```python
from build123d import *

# Parameters (mm, degrees)
SKETCH2_W           = 45
SKETCH2_H           = 10
BOSS_EXTRUDE1_DEPTH = 40
SKETCH4_W           = 45
SKETCH4_H           = 10
BOSS_EXTRUDE2_DEPTH = 10
SKETCH8_W           = 45
SKETCH8_H           = 10
BOSS_EXTRUDE3_DEPTH = 20
SKETCH9_R           = 1.45
CUT_EXTRUDE2_DEPTH  = 20
SKETCH10_W          = 45
SKETCH10_H          = 0.626165357
CUT_EXTRUDE3_DEPTH  = 2
SKETCH11_W          = 19
SKETCH11_H          = 42.671327575
BOSS_EXTRUDE4_DEPTH = 1.5
SKETCH12_W          = 3
SKETCH12_H          = 27.286335608
CUT_EXTRUDE6_DEPTH  = 10
SKETCH13_W          = 13
SKETCH13_H          = 22
BOSS_EXTRUDE5_DEPTH = 1


with BuildPart() as part:
    # Sketch2 → Boss-Extrude1 (new body)
    with BuildSketch(Plane(origin=(0, 0, 0), x_dir=(1, 0, 0), z_dir=(0, 1, 0))):
        Rectangle(SKETCH2_W, SKETCH2_H)
    extrude(amount=BOSS_EXTRUDE1_DEPTH)

    # Sketch4 → Boss-Extrude2 (add)
    with BuildSketch(Plane(origin=(0, 40, 0), x_dir=(1, 0, 0), z_dir=(0, 1, 0))):
        Rectangle(SKETCH4_W, SKETCH4_H)
    extrude(amount=BOSS_EXTRUDE2_DEPTH)

    # Sketch8 → Boss-Extrude3 (add)
    with BuildSketch(Plane.XZ):
        Rectangle(SKETCH8_W, SKETCH8_H)
    extrude(amount=BOSS_EXTRUDE3_DEPTH)

    # Sketch9 → Cut-Extrude2 (cut)
    with BuildSketch(Plane.XY.offset(5)):
        with Locations((19.5, 11.5)):
            Circle(SKETCH9_R)
        with Locations((-19.5, 11.5)):
            Circle(SKETCH9_R)
    extrude(amount=-CUT_EXTRUDE2_DEPTH, mode=Mode.SUBTRACT)

    # Sketch10 → Cut-Extrude3 (cut)
    with BuildSketch(Plane.XY.offset(5)):
        with Locations((0, 22.984410254)):
            Rectangle(SKETCH10_W, SKETCH10_H)
    extrude(amount=-CUT_EXTRUDE3_DEPTH, mode=Mode.SUBTRACT)

    # Sketch11 → Boss-Extrude4 (add)
    with BuildSketch(Plane.XY.offset(5)):
        with Locations((0, 1.335663788)):
            Rectangle(SKETCH11_W, SKETCH11_H)
    extrude(amount=BOSS_EXTRUDE4_DEPTH)

    # Sketch12 → Cut-Extrude6 (cut)
    with BuildSketch(Plane(origin=(22.5, 0, 0), x_dir=(0, 0, -1), z_dir=(1, 0, 0))):
        with Locations((0, -4.971840229)):
            Rectangle(SKETCH12_W, SKETCH12_H)
    cut_extrude6 = extrude(amount=-CUT_EXTRUDE6_DEPTH, mode=Mode.SUBTRACT)

    # Sketch13 → Boss-Extrude5 (add)
    with BuildSketch(Plane.XY.offset(5)):
        with Locations((16, -9)):
            Rectangle(SKETCH13_W, SKETCH13_H)
    boss_extrude5 = extrude(amount=BOSS_EXTRUDE5_DEPTH)

    # Mirror1: Cut-Extrude6 across plane
    add(cut_extrude6.mirror(Plane(origin=(0, 0, 0), x_dir=(0, 0, 1), z_dir=(1, 0, 0))), mode=Mode.SUBTRACT)

    # Mirror2: Boss-Extrude5 across plane
    add(boss_extrude5.mirror(Plane(origin=(0, 0, 0), x_dir=(0, 0, 1), z_dir=(1, 0, 0))))


solid = part.part
```
Geometry check sheet. Reference: the model listing, model coordinates, mm. A direction names the side the tool comes from. Coordinates: 2 decimals unless noted, no trailing zeros. Loops run counter-clockwise (first coordinate to the right, second up) from the corner with the lowest first, then second, coordinate; pieces in that order, holes last. Notation, with made-up numbers: (-14, 58) -> (38, 58) arc R12 ccw to (38, 66) -> close; hole circle Ø3 at (-21, 82). An arc over 180 degrees is marked (long way). Put each result on its own line as item: value.
1) Cross-section at C-C on y = 20.5. Record the boundary of the cut face in (x, z), plus the area to 4 significant figures.
Result set:
outline: (-22.5, -5) -> (22.5, -5) -> (22.5, 5) -> (9.5, 5) -> (9.5, 6.5) -> (-9.5, 6.5) -> (-9.5, 5) -> (-22.5, 5) -> close
area: 478.5 mm^2
2) Cross-section at D-D on x = -5. Record the boundary of the cut face in (y, z), plus the area to 3 significant figures.
Result set:
outline: (-20, -5) -> (50, -5) -> (50, 5) -> (23.3, 5) -> (23.3, 3) -> (22.67, 3) -> (22.67, 6.5) -> (-20, 6.5) -> close
area: 763 mm^2
3) Tool access check on faces 5 (the flat face through (16, -9, 6)), 6 (the flat face through (0, 23.297, 4)), 7 (the flat face through (-16, 12, 5)), 8 (the flat face through (-18, -5, -1.5)), 9 (the flat face through (18, 8.671, 0)). Record the directions out of +Z, -Z, +X, -X, +Y, -Y that give a thin tool (end or side, any length) a straight path to the whole face; none if there is none.
Result set:
face 5: +Z, +X, +Y, -Y
face 6: +Z, +X, -X
face 7: +Z, -X, +Y
face 8: -X
face 9: +X
4) Cross-section at A-A on x = 19.5. Count the separate pieces of the cut face and the enclosed holes in it, plus the area to 3 significant figures.
Result set:
separate pieces: 2
enclosed holes: 1
area: 610 mm^2
5) Cross-section at B-B on y = 11.5. Record the boundary of the cut face in (x, z), plus the area to 4 significant figures.
Result set:
outline: (-22.5, -5) -> (-20.95, -5) -> (-20.95, 5) -> (-22.5, 5) -> close; (-18.05, -5) -> (18.05, -5) -> (18.05, 5) -> (9.5, 5) -> (9.5, 6.5) -> (-9.5, 6.5) -> (-9.5, 5) -> (-18.05, 5) -> close; (20.95, -5) -> (22.5, -5) -> (22.5, 5) -> (20.95, 5) -> close
area: 420.5 mm^2
6) Gauge pin test, flat ends, axial feed: pin 1 Ø4.5 at (x, y) = (-19.5, 11.5) entering from +Z; pin 2 Ø8 at (x, y) = (-15.5, -7.5) entering from +Z; pin 3 Ø2.5 at (x, y) = (19.5, 11.5) entering from +Z; pin 4 Ø0.9 at (y, z) = (-10.5, -0.5) entering from +X. Record the tip position at first contact, or that the pin passes through.
Result set:
pin 1: stops at z = 5
pin 2: stops at z = 6
pin 3: passes through
pin 4: stops at x = 12.5
7) Thickness scan on line 1 (Y direction, x = -19.5, z = 0.25) (3 decimals); line 2 (Y direction, x = 16, z = -0.5) (3 decimals); line 3 (Z direction, x = 16.5, y = 5). Record the ranges inside material, lowest first.
Result set:
line 1: y = -20 to -18.615, 8.671 to 10.05, 12.95 to 50
line 2: y = -20 to -18.615, 8.671 to 50
line 3: z = -5 to -1.5, 1.5 to 5
8) Release check for a two-part mould opening along Y. For faces 1 (the flat face through (9.5, 6, 6)), 2 (the flat face through (-18, 8.671, 0)), 3 (the flat face through (0, 50, 0)), 4 (the flat face through (-12.5, -5, 0)) record: released by +Y, released by -Y, zero draft, split by the parting line, or undercut.
Result set:
face 1: zero draft
face 2: undercut
face 3: released by +Y
face 4: undercut
